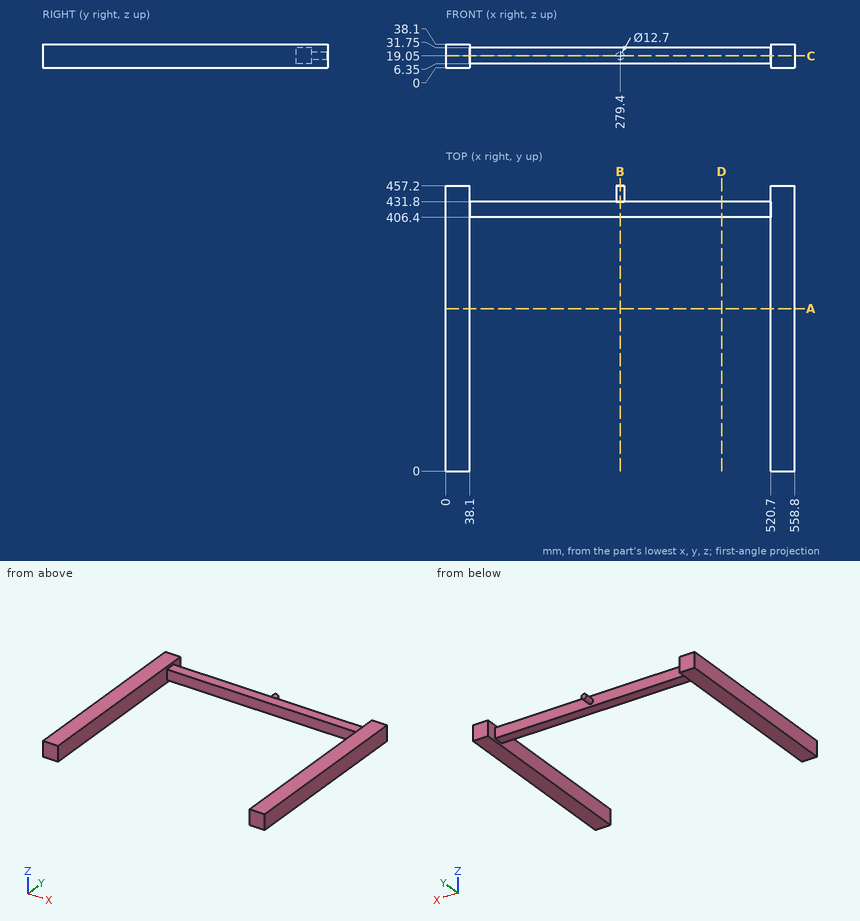
Study the drawing (mm; zero at the part's minimum x, y, z) and answer. Round coordinates to 2 decimals unless told otherwise and drop trailing zeros. Loops run counter-clockwise (first coordinate to the right, second up) from the corner with the lowest first, then second, coordinate; pieces in that order, holes last.
Q1. Section C-C, the plane z = 19.05 is taken. Determine the outline of the cut face in (x, y), then the cut area to 3 significant figures.
Q2. Section B-B, the plane x = 279.4 is taken. Determine the outline of the cut face in (y, z), then the cut area to 3 significant figures.
Q3. Section D-D, the plane x = 442 is taken. Determine the outline of the cut face in (y, z).
Q4. Find the intervals of material crossed by line 1 (X direction, y = 98, z = 12); line 2 (Z direction, x = 206.5, y = 423.5); line 3 (Y direction, x = 153, z = 14.5), in increasing order.
Q5. Section A-A, the plane y = 260.5 is taken. Determine the outline of the cut face in (x, z), then the cut area to 3 significant figures.
Q6. Given pin 1 Ø20.5 at (x, z) = (196, 18) entering from -Y; pin 2 Ø11.5 at (y, z) = (145, 11) entering from -X; pin 3 Ø1.5 at (x, z) = (215.5, 10) entering from +Y; pin 4 Ø12.5 at (x, y) = (235, 415) entering from +Z, each flat-ended and moving along its own axis, determine where each tip first touches the part or whether it passes through.
Completed:
1. outline: (0, 0) - (38.1, 0) - (38.1, 406.4) - (520.7, 406.4) - (520.7, 0) - (558.8, 0) - (558.8, 457.2) - (520.7, 457.2) - (520.7, 431.8) - (285.75, 431.8) - (285.75, 457.2) - (273.05, 457.2) - (273.05, 431.8) - (38.1, 431.8) - (38.1, 457.2) - (0, 457.2) - close
1. area: 47,400 mm2
2. outline: (406.4, 6.35) - (431.8, 6.35) - (431.8, 12.7) - (457.2, 12.7) - (457.2, 25.4) - (431.8, 25.4) - (431.8, 31.75) - (406.4, 31.75) - close
2. area: 968 mm2
3. outline: (406.4, 6.35) - (431.8, 6.35) - (431.8, 31.75) - (406.4, 31.75) - close
4. line 1: x = 0 to 38.1, 520.7 to 558.8
4. line 2: z = 6.35 to 31.75
4. line 3: y = 406.4 to 431.8
5. outline: (0, 0) - (38.1, 0) - (38.1, 38.1) - (0, 38.1) - close; (520.7, 0) - (558.8, 0) - (558.8, 38.1) - (520.7, 38.1) - close
5. area: 2,900 mm2
6. pin 1: stops at y = 406.4
6. pin 2: stops at x = 0
6. pin 3: stops at y = 431.8
6. pin 4: stops at z = 31.75
